Part model, mm, in its own coordinate system. A direction names the side the tool comes from. Round coordinates to 2 decimals unless told otherwise and drop trailing zeros. Write each loop counter-clockwise with the first axis right and the second up, starting at its lowest first coordinate (ties: lowest second). Pieces come first, ordered by that corner, then holes.
```python
from build123d import *

# Parameters (mm, degrees)
SKETCH1_W           = 83.722982013
SKETCH1_H           = 46.138643349
BOSS_EXTRUDE1_DEPTH = 4
SKETCH2_W           = 83.722982013
SKETCH2_H           = 4.859440563
BOSS_EXTRUDE2_DEPTH = 30
CUT_EXTRUDE10_DEPTH = 18
CUT_EXTRUDE11_DEPTH = 18
SKETCH7_W           = 22.745855452
SKETCH7_H           = 4
CUT_EXTRUDE14_DEPTH = 54
SKETCH8_W           = 11.05148618
SKETCH8_H           = 10.398194851
CUT_EXTRUDE15_DEPTH = 2
SKETCH9_W           = 9.731504247
SKETCH9_H           = 2.37712486
CUT_EXTRUDE16_DEPTH = 8
SKETCH10_W          = 2.06895071
SKETCH10_H          = 10.033558555
CUT_EXTRUDE17_DEPTH = 8
SKETCH11_W          = 1.186464173
SKETCH11_H          = 4
CUT_EXTRUDE18_DEPTH = 47
CUT_EXTRUDE19_DEPTH = 47
SKETCH13_R          = 1.414529115
CUT_EXTRUDE20_DEPTH = 58


with BuildPart() as part:
    # Sketch1 → Boss-Extrude1 (new body)
    with BuildSketch(Plane(origin=(0, 0, 0), x_dir=(1, 0, 0), z_dir=(0, 1, 0))):
        with Locations((41.861491007, 23.069321675)):
            Rectangle(SKETCH1_W, SKETCH1_H)
    extrude(amount=BOSS_EXTRUDE1_DEPTH)

    # Sketch2 → Boss-Extrude2 (add)
    with BuildSketch(Plane(origin=(0, 0, 0), x_dir=(1, 0, 0), z_dir=(0, 1, 0))):
        with Locations((41.861491007, 43.708923068)):
            Rectangle(SKETCH2_W, SKETCH2_H)
        with Locations((41.740293795, 2.496094928)):
            Rectangle(SKETCH2_W, SKETCH2_H)
    extrude(amount=BOSS_EXTRUDE2_DEPTH)

    # Sketch3 → Cut-Extrude10 (cut)
    with BuildSketch(Plane.XY.offset(-0.066374646)):
        Polygon((83.601784801, 30), (83.601784801, 4), (60.885327478, 4), align=None)
    extrude(amount=-CUT_EXTRUDE10_DEPTH, mode=Mode.SUBTRACT)

    # Sketch6 → Cut-Extrude11 (cut)
    with BuildSketch(Plane.XY.offset(-41.279202786)):
        Polygon((83.722982013, 30), (59.790662388, 4), (83.722982013, 4), align=None)
    extrude(amount=-CUT_EXTRUDE11_DEPTH, mode=Mode.SUBTRACT)

    # Sketch7 → Cut-Extrude14 (cut)
    with BuildSketch(Plane.XY):
        with Locations((72.350054287, 2)):
            Rectangle(SKETCH7_W, SKETCH7_H)
    extrude(amount=-CUT_EXTRUDE14_DEPTH, mode=Mode.SUBTRACT)

    # Sketch8 → Cut-Extrude15 (cut)
    with BuildSketch(Plane.XZ):
        with Locations((23.113449186, -14.294853075)):
            Rectangle(SKETCH8_W, SKETCH8_H)
    extrude(amount=-CUT_EXTRUDE15_DEPTH, mode=Mode.SUBTRACT)

    # Sketch9 → Cut-Extrude16 (cut)
    with BuildSketch(Plane.XY.offset(-0.066374646)):
        with Locations((13.369827145, 28.81143757)):
            Rectangle(SKETCH9_W, SKETCH9_H)
    extrude(amount=-CUT_EXTRUDE16_DEPTH, mode=Mode.SUBTRACT)

    # Sketch10 → Cut-Extrude17 (cut)
    with BuildSketch(Plane.XY.offset(-0.066374646)):
        with Locations((1.781804149, 16.215704525)):
            Rectangle(SKETCH10_W, SKETCH10_H)
    extrude(amount=-CUT_EXTRUDE17_DEPTH, mode=Mode.SUBTRACT)

    # Sketch11 → Cut-Extrude18 (cut)
    with BuildSketch(Plane(origin=(0, 0, -46.138643349), x_dir=(-1, 0, 0), z_dir=(0, 0, -1))):
        with Locations((-60.383894475, 2)):
            Rectangle(SKETCH11_W, SKETCH11_H)
    extrude(amount=-CUT_EXTRUDE18_DEPTH, mode=Mode.SUBTRACT)

    # Sketch12 → Cut-Extrude19 (cut)
    with BuildSketch(Plane(origin=(0, 0, -4.925815209), x_dir=(-1, 0, 0), z_dir=(0, 0, -1))):
        Polygon((-59.790662388, 4), (-83.478150153, 29.858494623), (-60.885327478, 4), align=None)
    extrude(amount=-CUT_EXTRUDE19_DEPTH, mode=Mode.SUBTRACT)

    # Sketch13 → Cut-Extrude20 (cut)
    with BuildSketch(Plane.XY.offset(-0.066374646)):
        with Locations((68.55855115, 27.64576808)):
            Circle(SKETCH13_R)
        with Locations((24.208487852, 28.064292507)):
            Circle(SKETCH13_R)
    extrude(amount=-CUT_EXTRUDE20_DEPTH, mode=Mode.SUBTRACT)


solid = part.part
```
Q1. Cut at C-C on z = -16. Write the cut outline in (x, y).
Values follow:
outline: (0, 0) - (17.59, 0) - (17.59, 2) - (28.64, 2) - (28.64, 0) - (59.79, 0) - (59.79, 4) - (0, 4) - close
Q2. Mould opens along X. For faces 1 (the flat face through (71.47, 16.75, -2.53)), 2 (the flat face through (23, 1, -19.494)), 3 (the flat face through (29, 0, -23)) say: +X half, -X half, draft (parallel to the pull), parting line (faces both ways), or undercut.
Values follow:
face 1: +X half
face 2: undercut
face 3: draft
Q3. Cut at D-D on y = 14. Write the cut outline in (x, z).
Values follow:
outline: (-0.12, -4.93) - (0.75, -4.93) - (0.75, -0.07) - (-0.12, -0.07) - close; (0, -46.14) - (69, -46.14) - (69, -41.28) - (0, -41.28) - close; (2.82, -4.93) - (68.95, -4.93) - (68.95, -0.07) - (2.82, -0.07) - close
Q4. Cut at A-A on y = 10. Write the cut outline in (x, z), plus the area to 3 significant figures.
Values follow:
outline: (-0.12, -4.93) - (65.29, -4.93) - (65.29, -0.07) - (-0.12, -0.07) - close; (0, -46.14) - (65.31, -46.14) - (65.31, -41.28) - (0, -41.28) - close
area: 635 mm2
Q5. Drop flat-ended pins along their axis: pin 1 (13 mm diameter, centred on x = 43.5, y = 14.5, fed in from +Z); pin 2 (11 mm diameter, centred on x = 15, z = -16.5, fed in from +Y); pin 3 (1.5 mm diameter, centred on x = 15, z = -3, fed in from +Y). Give the stop position or say it passes through.
Values follow:
pin 1: stops at z = -0.07
pin 2: stops at y = 4
pin 3: stops at y = 27.62
Q6. Which spindle directions (+Z, -Z, +X, -X, +Y, -Y) get a long thin tool onto all of the face, cutting with end or side? Do faces 4 (the flat face through (0.747, 16, -2)), 5 (the flat face through (32, 18, -0.066)), 6 (the flat face through (59.791, 2, -23)), 7 (the flat face through (32, 17, -41.279)), 8 (the flat face through (8.504, 29, -2)). Say none if no direction does.
Values follow:
face 4: +Z
face 5: +Z, +X, -X, +Y
face 6: +Z, -Z, +X, -Y
face 7: +X, -X, +Y
face 8: +Z, +Y
Q7. Cut at B-B on x = 64. Write the cut outline in (y, z).
Values follow:
outline: (8.57, -46.14) - (30, -46.14) - (30, -41.28) - (8.57, -41.28) - close; (8.6, -4.93) - (30, -4.93) - (30, -0.07) - (8.6, -0.07) - close
Q8. Wall check: L1, parallel to Z at x = 54, y = 19; L2, parallel to Y at x = 45, z = -40; L3, parallel to Y at x = 19.5, z = -15. Give the ranges that are in metal, low to high.
Values follow:
L1: z = -46.14 to -41.28, -4.93 to -0.07
L2: y = 0 to 4
L3: y = 2 to 4
